Check sheet for the modelled part. Datum: model origin and axes. Units: mm. Round coordinates to 2 decimals unless told otherwise and drop trailing zeros. Write each loop counter-clockwise with the first axis right and the second up, starting at its lowest first coordinate (ties: lowest second). Pieces come first, ordered by that corner, then holes.
Item 1: Depth check by flat-ended pin: pin 1 (3 mm diameter, centred on y = 32.5, z = 3.5, fed in from +X); pin 2 (2 mm diameter, centred on x = -54.5, z = 6, fed in from +Y); pin 3 (1.5 mm diameter, centred on x = -67.5, z = 1.5, fed in from -Y). Enter the tip coordinate at first touch or a pass-through.
Item 2: Release check for a two-part mould opening along Y. For faces 1 (the cylindrical face through (-72.884, 23.68, 3.451)), 2 (the flat face through (-60, 20, 7)), 3 (the cylindrical face through (-62.095, 23.205, 3.549)) record: pulls with the +Y half, pulls with the -Y half, needs draft (parallel to the pull), parting line crosses it, or undercut.
Item 3: Section check B-B, the plane y = 25. Record the cut outline in (x, z).
Item 4: Section check D-D, the plane y = 17.25. Record the cut outline in (x, z), plus the area to 3 significant figures.
Item 5: Section check C-C, the plane z = 5. Record the cut outline in (x, y).
Item 6: Section check A-A, the plane x = -58.75. Record the cut outline in (y, z), plus the area to 3 significant figures.
Item 7: Material ranges on line 1 along X through (y, z) = (21.5, 5.75); line 2 along X through (y, z) = (28, 6); line 3 along X through (y, z) = (24, 4.75), recorded low to high.
from build123d import *

# Parameters (mm, degrees)
SKETCH1_R           = 13
SKETCH1_R_2         = 1.5
BOSS_EXTRUDE1_DEPTH = 8
SKETCH2_R           = 2.2
CUT_EXTRUDE1_DEPTH  = 10
CUT_EXTRUDE2_DEPTH  = 1


with BuildPart() as part:
    # Sketch1 → Boss-Extrude1 (new body)
    with BuildSketch(Plane.XY):
        with Locations((-59.896810081, 23.108337223)):
            Circle(SKETCH1_R)
        with Locations((-59.896810081, 23.108337223)):
            Circle(SKETCH1_R_2, mode=Mode.SUBTRACT)
    extrude(amount=BOSS_EXTRUDE1_DEPTH)

    # Sketch2 → Cut-Extrude1 (cut)
    with BuildSketch(Plane.XY.offset(8)):
        with Locations((-59.896810081, 23.108337223)):
            Circle(SKETCH2_R)
    extrude(amount=-CUT_EXTRUDE1_DEPTH, mode=Mode.SUBTRACT)

    # Sketch4 → Cut-Extrude2 (cut)
    with BuildSketch(Plane.XY.offset(8)):
        Polygon((-73.325248838, 36.16514022), (-53.384391692, 38.140415901), (-46.517922759, 36.16514022), (-46.517922759, 9.754225618), (-73.325248838, 9.754225618), align=None)
    extrude(amount=-CUT_EXTRUDE2_DEPTH, mode=Mode.SUBTRACT)


solid = part.part
Values found:
1. pin 1: stops at x = -49.57
1. pin 2: stops at y = 35.34
1. pin 3: stops at y = 12.06
2. face 1: parting line crosses it
2. face 2: needs draft
2. face 3: undercut
3. outline: (-72.76, 0) - (-61.02, 0) - (-61.02, 7) - (-72.76, 7) - close; (-58.77, 0) - (-47.04, 0) - (-47.04, 7) - (-58.77, 7) - close
4. outline: (-71.5, 0) - (-48.29, 0) - (-48.29, 7) - (-71.5, 7) - close
4. area: 162 mm2
5. outline: circle Ø26 at (-59.9, 23.11); hole circle Ø4.4 at (-59.9, 23.11)
6. outline: (10.16, 0) - (21.23, 0) - (21.23, 7) - (10.16, 7) - close; (24.99, 0) - (36.06, 0) - (36.06, 7) - (24.99, 7) - close
6. area: 155 mm2
7. line 1: x = -72.8 to -61.4, -58.4 to -47
7. line 2: x = -71.94 to -47.85
7. line 3: x = -72.87 to -61.91, -57.89 to -46.93
